from build123d import *

# Parameters (mm, degrees)
F0_W      = 117.348
F0_H      = 63.5
F1_DEPTH  = 50.8
F2_W      = 35.052
F2_H      = 12.7
F3_DEPTH  = 117.349
F4_W      = 15.748
F4_H      = 38.1
F5_DEPTH  = 207
F6_DEPTH  = 117.349
F7_W      = 41.148
F7_H      = 25.4409682324
F8_DEPTH  = 35.053
F9_W      = 56.896
F9_H      = 12.7
F10_DEPTH = 50.801
F11_W     = 15.748
F11_H     = 12.7
F12_DEPTH = 117.349
F13_R     = 9.525
F14_DEPTH = 35.053


# Not quite as in the source:
# - an extrude ends at something that could not be found from the text; its depth is read off the source's solid


with BuildPart() as f1:
    # F0 (on Front) → F1 (new body)
    with BuildSketch(Plane.XZ):
        Rectangle(F0_W, F0_H)
    extrude(amount=F1_DEPTH)

    # F2 (on face) → F3 (cut, through all)
    with BuildSketch(Plane(origin=(-58.674, 0, 0), x_dir=(0, -1, 0), z_dir=(-1, 0, 0))):
        with Locations((33.274, 25.4)):
            Rectangle(F2_W, F2_H)
    extrude(amount=-F3_DEPTH, mode=Mode.SUBTRACT)

    # F4 (on face) → F5 (cut, through all)
    with BuildSketch(Plane.YZ.offset(58.674)):
        with Locations((-42.926, 0)):
            Rectangle(F4_W, F4_H)
    extrude(amount=F5_DEPTH, mode=Mode.SUBTRACT)

    # F4 (on face) → F6 (cut, through all)
    with BuildSketch(Plane.YZ.offset(58.674)):
        with Locations((-42.926, 0)):
            Rectangle(F4_W, F4_H)
    extrude(amount=-F6_DEPTH, mode=Mode.SUBTRACT)

    # F7 (on face) → F8 (cut, through all)
    with BuildSketch(Plane.XZ.offset(35.052)):
        with Locations((38.1, 19.3680736702)):
            Rectangle(F7_W, F7_H)
    extrude(amount=-F8_DEPTH, mode=Mode.SUBTRACT)

    # F9 (on face) → F10 (cut, through all)
    with BuildSketch(Plane.XZ.offset(50.8)):
        with Locations((-30.226, -25.4)):
            Rectangle(F9_W, F9_H)
    extrude(amount=-F10_DEPTH, mode=Mode.SUBTRACT)

    # F11 (on face) → F12 (cut, through all)
    with BuildSketch(Plane.YZ.offset(58.674)):
        with Locations((-7.874, -25.4)):
            Rectangle(F11_W, F11_H)
    extrude(amount=-F12_DEPTH, mode=Mode.SUBTRACT)

    # F13 (on face) → F14 (cut, through all)
    with BuildSketch(Plane.XZ.offset(35.052)):
        with Locations((-38.413323462, -0.254)):
            Circle(F13_R)
    extrude(amount=-F14_DEPTH, mode=Mode.SUBTRACT)


solid = f1.part
Design review of the part built by this model. Coordinates are the model's own, in mm. A direction names the side the tool comes from. Coordinates: 2 decimals unless noted, no trailing zeros. Order: outer loops, then holes, each group sorted by start corner. A loop starts at its lowest first (then second) coordinate and runs counter-clockwise, first axis right, second up.
Item 1: For pin 1 Ø19 at (x, z) = (16, 2.5) entering from -Y; pin 2 Ø17 at (x, z) = (-38.41, -0.25) entering from +Y; pin 3 Ø9.5 at (x, y) = (-15, -28.5) entering from +Z; pin 4 Ø10.5 at (x, y) = (40, -12) entering from +Z, all flat-tipped, find the tip position at first contact; note any pin that passes through.
Item 2: Take a section at A-A, the plane x = -38. Write out the cut boundary in (y, z), then the cut area to 3 significant figures.
Item 3: For faces 1 (the flat face through (17.526, -14, 16)), 2 (the flat face through (29, -15.748, -25)), 3 (the flat face through (-21, -25, 19.05)), list the 3-axis set-ups (+Z, -Z, +X, -X, +Y, -Y) from which the entire face can be reached by the end or side of a thin tool; tool diameter is ignored.
Item 4: The part is to be moulded in two halves that separate along X. For faces 4 (the cylindrical face through (-29.615, -17.771, -3.902)), 5 (the flat face through (-1.778, -34, -25)), 6 (the flat face through (38, -18, 6.648)), say which applies: pulls with the +X half, pulls with the -X half, needs draft (parallel to the pull), parting line crosses it, or undercut.
Item 5: Take a section at C-C, the plane x = 7.5. Write out the cut boundary in (y, z).
Item 6: Take a section at B-B, the plane y = -10.5. Write out the cut boundary in (x, z) (3 decimals).
Item 7: Take a section at D-D, the plane z = 3.5. Write out the cut boundary in (x, y), then the cut area to 3 significant figures.
Item 8: For line 1 (Z direction, x = 19.5, y = -18); line 2 (Y direction, x = 4, z = 27.5); line 3 (Y direction, x = 36, z = 5.5), list the stretches that pass through material, from the lowest coordinate up.
The answers:
1. pin 1: stops at y = -35.05
1. pin 2: passes through
1. pin 3: stops at z = 19.05
1. pin 4: stops at z = 6.65
2. outline: (-35.05, -19.05) - (0, -19.05) - (0, -9.77) - (-35.05, -9.77) - close; (-35.05, 9.26) - (0, 9.26) - (0, 31.75) - (-15.75, 31.75) - (-15.75, 19.05) - (-35.05, 19.05) - close
2. area: 868 mm2
3. face 1: +Z, +X, +Y, -Y
3. face 2: -Z, +X, -X, +Y
3. face 3: +Z, +X, -X, -Y
4. face 4: undercut
4. face 5: pulls with the -X half
4. face 6: needs draft
5. outline: (-50.8, -31.75) - (-15.75, -31.75) - (-15.75, -19.05) - (0, -19.05) - (0, 31.75) - (-15.75, 31.75) - (-15.75, 19.05) - (-35.05, 19.05) - (-35.05, -19.05) - (-50.8, -19.05) - close
6. outline: (-58.674, -19.05) - (58.674, -19.05) - (58.674, 6.648) - (17.526, 6.648) - (17.526, 31.75) - (-58.674, 31.75) - close; hole circle Ø19.05 at (-38.413, -0.254)
7. outline: (-58.67, -35.05) - (-47.17, -35.05) - (-47.17, 0) - (-58.67, 0) - close; (-29.66, -35.05) - (58.67, -35.05) - (58.67, 0) - (-29.66, 0) - close
7. area: 3,500 mm2
8. line 1: z = -31.75 to 6.65
8. line 2: y = -15.75 to 0
8. line 3: y = -35.05 to 0
